Geometry: final body of the model. Coordinates: model frame, mm. A direction names the side the tool comes from. Coordinates: 2 decimals unless noted, no trailing zeros. Order: outer loops, then holes, each group sorted by start corner. A loop starts at its lowest first (then second) coordinate and runs counter-clockwise, first axis right, second up. Notation, with made-up numbers: M 70,80 L 79,80 A23 cw 79,95 Z; hole C 22.25,48.25 d4. An arc over 180 degrees is marked long. One line per question, with ' | ' between items.
from build123d import *

# Parameters (mm, degrees)
PAD007_DEPTH             = 2.7
CLONE087_ROLL_ANGLE      = 180
CYLINDER1014_R           = 2.7
CYLINDER1014_DEPTH       = 100
CYLINDER1018_R           = 1.7
CYLINDER1018_DEPTH       = 10
CLONE086_PITCH_ANGLE     = -90
CLONE086_PLACEMENT_ANGLE = -180
BOX044_W                 = 6
BOX044_H                 = 30
BOX044_DEPTH             = 15
CHAMFER017_SIZE          = 6
CYLINDER1039_R           = 10
CYLINDER1039_DEPTH       = 10
FILLET_R                 = 1


with BuildPart() as clone_of_m3nuthousingmaster012:
    # Sketch008 → Pad007 (new body)
    with BuildSketch(Plane(origin=(65, 30, 1.5), x_dir=(0, 0, 1), z_dir=(-1, 0, 0))):
        Polygon((0, 0), (1.674316, 2.9), (21.674316, 2.9), (21.674316, -2.9), (1.674316, -2.9), align=None)
    extrude(amount=PAD007_DEPTH)


with BuildPart() as clone_of_m3nuthousingmaster012_1:
    # Clone087 roll: moved
    add(clone_of_m3nuthousingmaster012.part.rotate(Axis((0, 0, 0), (1, 0, 0)), CLONE087_ROLL_ANGLE))


with BuildPart() as clone_of_m3nuthousingmaster012_2:
    # Clone087 placement: moved
    add(clone_of_m3nuthousingmaster012_1.part.moved(Location((-58.3, 30, 10))))


with BuildPart() as obj1:
    # Cylinder1014 → Cylinder1014 (new body)
    with BuildSketch(Plane.XY):
        Circle(CYLINDER1014_R)
    extrude(amount=CYLINDER1014_DEPTH)


with BuildPart() as obj1_1:
    # Clone085 placement: moved
    add(obj1.part.moved(Location((0, 0, -90))))


with BuildPart() as fusion069:
    # Cylinder1018 → Cylinder1018 (new body)
    with BuildSketch(Plane.XY):
        Circle(CYLINDER1018_R)
    extrude(amount=CYLINDER1018_DEPTH)


with BuildPart() as fusion069_1:
    # Clone086 pitch: moved
    add(fusion069.part.rotate(Axis((0, 0, 0), (0, 1, 0)), CLONE086_PITCH_ANGLE))


with BuildPart() as fusion069_2:
    # Clone086 placement: moved
    add(fusion069_1.part.moved(Location((1, 0, 5))).rotate(Axis((1, 0, 5), (0, 0, 1)), CLONE086_PLACEMENT_ANGLE))

    # Fusion069: union Clone of M3NutHousingMaster012, obj1
    add(clone_of_m3nuthousingmaster012_2.part)
    add(obj1_1.part)


with BuildPart() as chamfer017:
    # Box044 → Box044 (new body)
    with BuildSketch(Plane(origin=(-3, -15, 10), x_dir=(1, 0, 0), z_dir=(0, 0, 1))):
        with Locations((3, 15)):
            Rectangle(BOX044_W, BOX044_H)
    extrude(amount=BOX044_DEPTH)

    # Chamfer017
    chamfer017_edges = [chamfer017.edges().sort_by_distance(p)[0] for p in [
        (0, -15, 10),
        (0, -15, 25),
        (0, 15, 10),
        (0, 15, 25),
    ]]
    chamfer(chamfer017_edges, length=CHAMFER017_SIZE)


with BuildPart() as adjustwheel:
    # Cylinder1039 → Cylinder1039 (new body)
    with BuildSketch(Plane.XY):
        Circle(CYLINDER1039_R)
    extrude(amount=CYLINDER1039_DEPTH)

    # Fusion070: union Chamfer017
    add(chamfer017.part)

    # Fillet
    fillet_edges = [adjustwheel.edges().sort_by_distance(p)[0] for p in [
        (-10, 0, 10),
    ]]
    fillet(fillet_edges, radius=FILLET_R)

    # Cut052: cut Fusion069
    add(fusion069_2.part, mode=Mode.SUBTRACT)


solid = adjustwheel.part
1. Section B-B, the plane z = 19.75. Output: boundary loops of the cut face in (x, y), and give its area (3 significant figures).
Response values:
outline: M -3,-14.25 L 3,-14.25 L 3,14.25 L -3,14.25 Z | area: 171 mm^2
2. Section A-A, the plane z = 2.5. Output: boundary loops of the cut face in (x, y).
Response values:
outline: C 0,0 d20; hole C 0,0 d5.4; hole M 4,-2.9 L 6.7,-2.9 L 6.7,2.9 L 4,2.9 Z
3. Section C-C, the plane z = 5.25. Output: boundary loops of the cut face in (x, y), and give its area (3 significant figures).
Response values:
outline: M 2.11,-1.68 A2.7 cw long 2.11,1.68 L 4,1.68 L 4,2.9 L 6.7,2.9 L 6.7,1.68 L 9.86,1.68 A10 ccw long 9.86,-1.68 L 6.7,-1.68 L 6.7,-2.9 L 4,-2.9 L 4,-1.68 Z | area: 260 mm^2
4. Pin query (flat end, axial travel): P1, Ø12, axis at x = 6.5, z = 5.5, coming from the -Y side; P2, Ø6, axis at x = 7.5, y = -7.5, coming from the +Z side; P3, Ø4, axis at y = 0, z = 5, coming from the +X side; P4, Ø2, axis at x = 6, z = 4, coming from the +Y side. Return the tip coordinate at first contact, or that it passes through.
Response values:
P1: stops at y = -9.99 | P2: stops at z = 10 | P3: stops at x = 10 | P4: stops at y = 8.66
5. Material intervals for line 1 (X direction, y = 0, z = 3); line 2 (Y direction, x = 0, z = 4); line 3 (X direction, y = 1, z = 2.5), sorted ascending. Write a range as [from, to].
Response values:
line 1: x = [-10, -2.7], [2.7, 4], [6.7, 10] | line 2: y = [-10, -2.7], [2.7, 10] | line 3: x = [-9.95, -2.51], [2.51, 4], [6.7, 9.95]
6. Access query for faces 1 (the face through (8.33, 0.65, 6.57)), 2 (the face through (5.369, -1.43, 7.675)), 3 (the face through (3, 0, 17)), 4 (the face through (-3, 0, 17)). Directions: +Z, -Z, +X, -X, +Y, -Y. A direction counts if a zero-diameter tool reaches every point of the face in a straight line with its end or side. Return the directions, or none.
Response values:
face 1: +X | face 2: -Z | face 3: +Z, +X, +Y, -Y | face 4: +Z, -X, +Y, -Y
7. Draft query along Z for faces 5 (the face through (3.25, -0.07, 3.3)), 6 (the face through (-5, 0, 10)), 7 (the face through (4, 0, 3)). Return one class per face: pulls with the +Z half, pulls with the -Z half, needs draft (parallel to the pull), parting line crosses it, or undercut.
Response values:
face 5: undercut | face 6: pulls with the +Z half | face 7: needs draft
